Design review of the part built by this model. Coordinates are the model's own, in mm. Face numbers are marked on the shaded views. A direction names the side the tool comes from. Coordinates: 2 decimals unless noted, no trailing zeros. Write each loop counter-clockwise with the first axis right and the second up, starting at its lowest first coordinate (ties: lowest second). Pieces come first, ordered by that corner, then holes.
Q1. Take a section at D-D (y = 8.75). Give the boundary of the cut face in (x, z) (3 decimals), and give its area (3 significant figures).
Q2. Take a section at B-B (y = 6). Give the boundary of the cut face in (x, z), and give its area (3 significant figures).
Q3. Mouldability with a two-part tool opening along Z and no side actions: class the marked faces 1, 2 and 3 as pulls with the +Z half, pulls with the -Z half, needs draft (parallel to the pull), parting line crosses it, or undercut.
Q4. Take a section at C-C (y = 11.25). Give the boundary of the cut face in (x, z), and give its area (3 significant figures).
Q5. Take a section at A-A (y = 3.5). Give the boundary of the cut face in (x, z), and give its area (3 significant figures).
Q6. For probe 1 along Z at (x, y) = (0, 6.5); probe 2 along Z at (x, y) = (0, 3.5); probe 3 along X at (y, z) = (6.5, 1), list the stretches that pass through material, from the lowest coordinate up.
Q7. Machinability: for the marked faces 4, 5 and 6, which of the approach directions +Z, -Z, +X, -X, +Y, -Y give a long, thin tool a straight path to every point of the face, cutting with its end or side? Answer none if there is none.
Q8. Insertion check: pin 1 (1.5 mm diameter, centred on x = 3.5, z = 2, fed in from +Y); pin 2 (1 mm diameter, centred on x = 2.5, z = -0.5, fed in from -Y); pin 3 (1 mm diameter, centred on x = -3, z = 1.5, fed in from +Y). Each pin has a flat end and moves straight along its axis. Give the tip position at first contact, or say it passes through.
```python
from build123d import *

# Parameters (mm, degrees)
SKETCH_2_OUTSIDE_W  = 17.542
SKETCH_2_OUTSIDE_H  = 17.542
CUT_EXTRUDE_1_DEPTH = 15.495689014
CHAMFER_1_SIZE      = 0.6


with BuildPart() as part:
    # Эскиз1 → Revolve 782 (revolve)
    with BuildSketch(Plane.XY, mode=Mode.PRIVATE) as revolve_782_sk:
        with BuildLine():
            Line((5.75, 0.577350269), (5.75, 4.422649731))
            Line((5.75, 4.422649731), (4.75, 5))
            Line((4.75, 5), (4.75, 7.25))
            ThreePointArc((4.75, 7.25), (3.358757211, 10.608757211), (0, 12))
            Line((0, 12), (0, 10))
            Line((0, 10), (2.6, 8))
            Line((2.6, 8), (2.6, 0))
            Line((2.6, 0), (4.75, 0))
            Line((4.75, 0), (5.75, 0.577350269))
        make_face()
    revolve(revolve_782_sk.sketch.rotate(Axis((0, 18.372325569, 0), (0, -1, 0)), 180), axis=Axis((0, 18.372325569, 0), (0, -1, 0)))

    # Эскиз2 outside → Вырез-Вытянуть1 (cut, through all)
    with BuildSketch(Plane(origin=(0, 0, 0), x_dir=(1, 0, 0), z_dir=(0, 1, 0))):
        Rectangle(SKETCH_2_OUTSIDE_W, SKETCH_2_OUTSIDE_H)
        Polygon((0, 5.773502692), (-5, 2.886751346), (-5, -2.886751346), (0, -5.773502692), (5, -2.886751346), (5, 2.886751346), align=None, mode=Mode.SUBTRACT)
    extrude(amount=CUT_EXTRUDE_1_DEPTH, mode=Mode.SUBTRACT)

    # Фаска1
    chamfer_1_edges = [part.edges().sort_by_distance(p)[0] for p in [
        (2.6, 0, 0),
    ]]
    chamfer(chamfer_1_edges, length=CHAMFER_1_SIZE)


solid = part.part
```
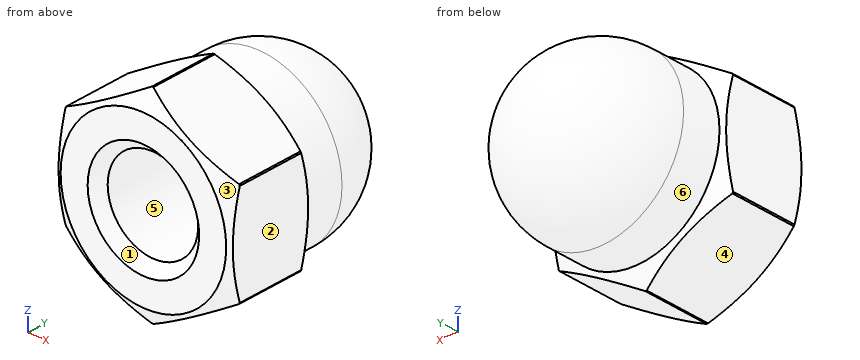
Response:
1. outline: circle Ø9.014 at (0, 0); hole circle Ø3.25 at (0, 0)
1. area: 55.5 mm2
2. outline: circle Ø9.5 at (0, 0); hole circle Ø5.2 at (0, 0)
2. area: 49.6 mm2
3. face 1: undercut
3. face 2: needs draft
3. face 3: parting line crosses it
4. outline: circle Ø5.12 at (0, 0)
4. area: 20.6 mm2
5. outline: (-5, -2.84) arc R5.75 ccw to (-4.96, -2.91) - (-0.04, -5.75) arc R5.75 ccw to (0.04, -5.75) - (4.96, -2.91) arc R5.75 ccw to (5, -2.84) - (5, 2.84) arc R5.75 ccw to (4.96, 2.91) - (0.04, 5.75) arc R5.75 ccw to (-0.04, 5.75) - (-4.96, 2.91) arc R5.75 ccw to (-5, 2.84) - close; hole circle Ø5.2 at (0, 0)
5. area: 65.4 mm2
6. probe 1: z = -4.75 to -2.6, 2.6 to 4.75
6. probe 2: z = -5.75 to -2.6, 2.6 to 5.75
6. probe 3: x = -4.64 to -2.4, 2.4 to 4.64
7. face 4: -Z, -X, +Y, -Y
7. face 5: -Y
7. face 6: +Y
8. pin 1: stops at y = 10.68
8. pin 2: stops at y = 0.15
8. pin 3: stops at y = 11.05
